from build123d import *

# Parameters (mm, degrees)
PAD038_DEPTH    = 80
POCKET025_DEPTH = 11.4010000384
POCKET026_DEPTH = 11.4010366708


with BuildPart() as part:
    # Sketch063 (on Face65 of Binder012) → Pad038 (new body)
    with BuildSketch(Plane.XY.offset(9.8)):
        Polygon((-93.5396103068, 82.1395919522), (-85.1396103452, 82.1395919522), (-85.1396103452, 73.7395919906), (-82.1396102684, 73.7395919906), (-82.1396102684, 82.1395919522), (-73.7396103068, 82.1396286614), (-73.7396103068, 85.1396286614), (-82.1396102684, 85.1396286614), (-82.1396103452, 93.539628623), (-85.1396103452, 93.539628623), (-85.1396103452, 85.1396286614), (-93.5396103068, 85.1396286614), align=None)
    extrude(amount=PAD038_DEPTH)

    # Sketch064 (on Face2 of Pad038) → Pocket025 (cut, through all)
    with BuildSketch(Plane(origin=(-85.1396103452, 0, 0), x_dir=(0, -1, 0), z_dir=(-1, 0, 0))):
        Polygon((-87.1396286614, 13.5071067812), (-87.1396286614, 15.0928932188), (-87.8467354426, 15.8), (-89.4325218802, 15.8), (-90.1396286614, 15.0928932188), (-90.1396286614, 13.5071067812), (-89.4325218802, 12.8), (-87.8467354426, 12.8), align=None)
        Polygon((-79.432485171, 12.8), (-77.8466987333, 12.8), (-77.1395919522, 13.5071067812), (-77.1395919522, 15.0928932188), (-77.8466987333, 15.8), (-79.432485171, 15.8), (-80.1395919522, 15.0928932188), (-80.1395919522, 13.5071067812), align=None)
        Polygon((-89.4325218802, 20.8), (-87.8467354426, 20.8), (-87.1396286614, 21.5071067812), (-87.1396286614, 23.0928932188), (-87.8467354426, 23.8), (-89.4325218802, 23.8), (-90.1396286614, 23.0928932188), (-90.1396286614, 21.5071067812), align=None)
        Polygon((-79.432485171, 20.8), (-77.8466987333, 20.8), (-77.1395919522, 21.5071067812), (-77.1395919522, 23.0928932188), (-77.8466987333, 23.8), (-79.432485171, 23.8), (-80.1395919522, 23.0928932188), (-80.1395919522, 21.5071067812), align=None)
        Polygon((-90.1396286614, 86.0928932188), (-90.1396286614, 84.5071067812), (-89.4325218802, 83.8), (-87.8467354426, 83.8), (-87.1396286614, 84.5071067812), (-87.1396286614, 86.0928932188), (-87.8467354426, 86.8), (-89.4325218802, 86.8), align=None)
        Polygon((-80.1395919522, 86.0928932188), (-80.1395919522, 84.5071067812), (-79.432485171, 83.8), (-77.8466987333, 83.8), (-77.1395919522, 84.5071067812), (-77.1395919522, 86.0928932188), (-77.8466987333, 86.8), (-79.432485171, 86.8), align=None)
        Polygon((-90.1396286614, 78.0928932188), (-90.1396286614, 76.5071067812), (-89.4325218802, 75.8), (-87.8467354426, 75.8), (-87.1396286614, 76.5071067812), (-87.1396286614, 78.0928932188), (-87.8467354426, 78.8), (-89.4325218802, 78.8), align=None)
        Polygon((-80.1395919522, 78.0928932188), (-80.1395919522, 76.5071067812), (-79.432485171, 75.8), (-77.8466987333, 75.8), (-77.1395919522, 76.5071067812), (-77.1395919522, 78.0928932188), (-77.8466987333, 78.8), (-79.432485171, 78.8), align=None)
    extrude(amount=-POCKET025_DEPTH, mode=Mode.SUBTRACT)

    # Sketch065 (on Face6 of Pocket025) → Pocket026 (cut, through all)
    with BuildSketch(Plane(origin=(0, 85.1396286614, 0), x_dir=(-1, 0, 0), z_dir=(0, 1, 0))):
        Polygon((87.1396103452, 15.0928932188), (87.1396103452, 13.5071067812), (87.8467171264, 12.8), (89.432503564, 12.8), (90.1396103452, 13.5071067812), (90.1396103452, 15.0928932188), (89.432503564, 15.8), (87.8467171264, 15.8), align=None)
        Polygon((87.1396103452, 23.0928932188), (87.1396103452, 21.5071067812), (87.8467171264, 20.8), (89.432503564, 20.8), (90.1396103452, 21.5071067812), (90.1396103452, 23.0928932188), (89.432503564, 23.8), (87.8467171264, 23.8), align=None)
        Polygon((79.4325034872, 15.8), (77.8467170496, 15.8), (77.1396102684, 15.0928932188), (77.1396102684, 13.5071067812), (77.8467170496, 12.8), (79.4325034872, 12.8), (80.1396102684, 13.5071067812), (80.1396102684, 15.0928932188), align=None)
        Polygon((79.4325034872, 23.8), (77.8467170496, 23.8), (77.1396102684, 23.0928932188), (77.1396102684, 21.5071067812), (77.8467170496, 20.8), (79.4325034872, 20.8), (80.1396102684, 21.5071067812), (80.1396102684, 23.0928932188), align=None)
        Polygon((77.1396102684, 86.0928932188), (77.1396102684, 84.5071067812), (77.8467170496, 83.8), (79.4325034872, 83.8), (80.1396102684, 84.5071067812), (80.1396102684, 86.0928932188), (79.4325034872, 86.8), (77.8467170496, 86.8), align=None)
        Polygon((87.1396103452, 86.0928932188), (87.1396103452, 84.5071067812), (87.8467171264, 83.8), (89.432503564, 83.8), (90.1396103452, 84.5071067812), (90.1396103452, 86.0928932188), (89.432503564, 86.8), (87.8467171264, 86.8), align=None)
        Polygon((77.1396102684, 78.0928932188), (77.1396102684, 76.5071067812), (77.8467170496, 75.8), (79.4325034872, 75.8), (80.1396102684, 76.5071067812), (80.1396102684, 78.0928932188), (79.4325034872, 78.8), (77.8467170496, 78.8), align=None)
        Polygon((87.1396103452, 78.0928932188), (87.1396103452, 76.5071067812), (87.8467171264, 75.8), (89.432503564, 75.8), (90.1396103452, 76.5071067812), (90.1396103452, 78.0928932188), (89.432503564, 78.8), (87.8467171264, 78.8), align=None)
    extrude(amount=-POCKET026_DEPTH, mode=Mode.SUBTRACT)


solid = part.part
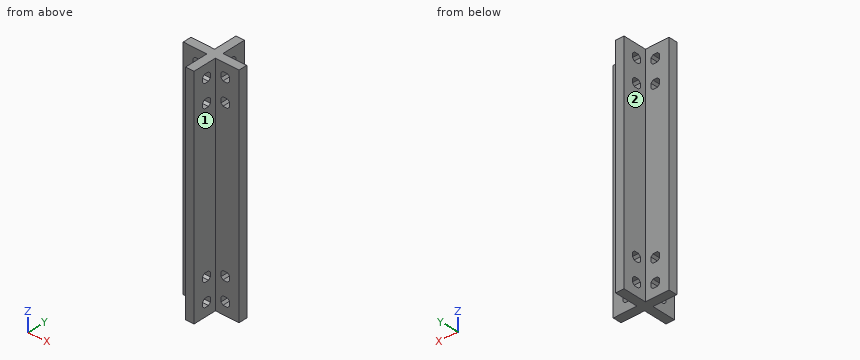
Verification items for the finished model (mm, model axes). Face numbers are marked on the shaded views. A direction names the side the tool comes from. Coordinates: 2 decimals unless noted, no trailing zeros. Write each loop counter-clockwise with the first axis right and the second up, starting at its lowest first coordinate (ties: lowest second). Pieces come first, ordered by that corner, then holes. Notation, with made-up numbers: M 6,45.5 L 46,45.5 A23 cw 46,63.5 Z; hole C -39,75 d8. An arc over 180 degrees is marked long. Use a Markdown table: item, result.
Q1. Sectioned sample at C-C, the plane z = 25. Record the boundary of the cut face in (x, y).
Reply:
| item | result |
|---|---|
| outline | M -93.54,82.14 L -85.14,82.14 L -85.14,73.74 L -82.14,73.74 L -82.14,82.14 L -73.74,82.14 L -73.74,85.14 L -82.14,85.14 L -82.14,93.54 L -85.14,93.54 L -85.14,85.14 L -93.54,85.14 Z |
Q2. Sectioned sample at D-D, the plane y = 91.25. Record the boundary of the cut face in (x, z).
Reply:
| item | result |
|---|---|
| outline | M -85.14,9.8 L -82.14,9.8 L -82.14,89.8 L -85.14,89.8 Z |
Q3. Go/stop test with flat-tipped pins: P1, Ø1, axis at x = -86, y = 76, coming from the +Z side; P2, Ø10, axis at x = -88.5, y = 77.5, coming from the -Z side; P3, Ø6.5, axis at y = 89.5, z = 55, coming from the -X side. Record where each tip stops, or that it passes through.
Reply:
| item | result |
|---|---|
| P1 | passes through |
| P2 | stops at z = 9.8 |
| P3 | stops at x = -85.14 |
Q4. Set-up check for the marked faces 1 and 2: record each of +Z, -Z, +X, -X, +Y, -Y from which the full face is reachable in a straight line by a thin tool's end or side.
Reply:
| item | result |
|---|---|
| face 1 | +Z, -Z, +X, -Y |
| face 2 | +Z, -Z, -X, +Y |
Q5. Sectioned sample at B-B, the plane x = -88.75. Record the boundary of the cut face in (y, z).
Reply:
| item | result |
|---|---|
| outline | M 82.14,9.8 L 85.14,9.8 L 85.14,12.8 L 82.14,12.8 Z; M 82.14,15.8 L 85.14,15.8 L 85.14,20.8 L 82.14,20.8 Z; M 82.14,23.8 L 85.14,23.8 L 85.14,75.8 L 82.14,75.8 Z; M 82.14,78.8 L 85.14,78.8 L 85.14,83.8 L 82.14,83.8 Z; M 82.14,86.8 L 85.14,86.8 L 85.14,89.8 L 82.14,89.8 Z |
Q6. Sectioned sample at A-A, the plane y = 78.75. Record the boundary of the cut face in (x, z), plus the area to 3 significant figures.
Reply:
| item | result |
|---|---|
| outline | M -85.14,9.8 L -82.14,9.8 L -82.14,12.8 L -85.14,12.8 Z; M -85.14,15.8 L -82.14,15.8 L -82.14,20.8 L -85.14,20.8 Z; M -85.14,23.8 L -82.14,23.8 L -82.14,75.8 L -85.14,75.8 Z; M -85.14,78.8 L -82.14,78.8 L -82.14,83.8 L -85.14,83.8 Z; M -85.14,86.8 L -82.14,86.8 L -82.14,89.8 L -85.14,89.8 Z |
| area | 204 mm² |
Q7. Thickness scan on line 1 (Z direction, x = -78.25, y = 82.25); line 2 (X direction, y = 87.5, z = 15.5); line 3 (Y direction, x = -81.75, z = 49). Record the ranges inside material, lowest first.
Reply:
| item | result |
|---|---|
| line 1 | z = 9.8 to 12.8, 15.8 to 20.8, 23.8 to 75.8, 78.8 to 83.8, 86.8 to 89.8 |
| line 2 | x = -85.14 to -82.14 |
| line 3 | y = 82.14 to 85.14 |
